Build history of the part. All positions in model axes, mm. Round coordinates to 2 decimals unless told otherwise and drop trailing zeros. Write each loop counter-clockwise with the first axis right and the second up, starting at its lowest first coordinate (ties: lowest second). Pieces come first, ordered by that corner, then holes.
Autodesk Inventor part; units mm, degrees
ref_plane "YZ Plane" through (0, 0, 0) normal (1, 0, 0) x (0, 1, 0)
ref_plane "XZ Plane" through (0, 0, 0) normal (0, 1, 0) x (-1, 0, 0)
ref_plane "XY Plane" through (0, 0, 0) normal (0, 0, 1) x (1, 0, 0)
sketch "Sketch1" plane through (0, 0, 0) normal (0, 1, 0) x (-1, 0, 0)
  line L0 (110, -15) -> (-110, -15)
  line L1 (-110, -15) -> (-110, 15)
  line L2 (-110, 15) -> (110, 15)
  line L3 (110, 15) -> (110, -15)
  line L4 (110, 0) -> (-110, 0) construction
  line L5 (0, -15) -> (0, 15) construction
  point P0 (0, 0)
  point P1 (0, 0)
  dimension "d0" = 220
  dimension "d1" = 30
extrude "Extrusion1" add sketch "Sketch1" along normal blind 15
sketch "Sketch2" plane through (-110, 0, -15) normal (-1, 0, 0) x (0, 0, 1)
  circle A0 centre (5, 7.5) radius 2.5
  line L0 (0, 0) -> (0, 15) construction
  line L1 (0, 7.5) -> (30, 7.5) construction
  line L2 (30, 0) -> (30, 15) construction
  line L3 (15, 0) -> (15, 15) construction
  line L4 (30, 15) -> (0, 15) construction
  circle A1 centre (25, 7.5) radius 2.5
  dimension "d4" = 5
  dimension "d5" = 20
extrude "Extrusion2" cut sketch "Sketch2" against normal blind 8
sketch "Sketch3" plane through (110, 0, 15) normal (1, 0, 0) x (0, 0, -1)
  circle A0 centre (25, 7.5) radius 2.5
  circle A1 centre (5, 7.5) radius 2.5
  point P0 (15, 0)
extrude "Extrusion3" cut sketch "Sketch3" against normal blind 8
properties part number "aux_strut"
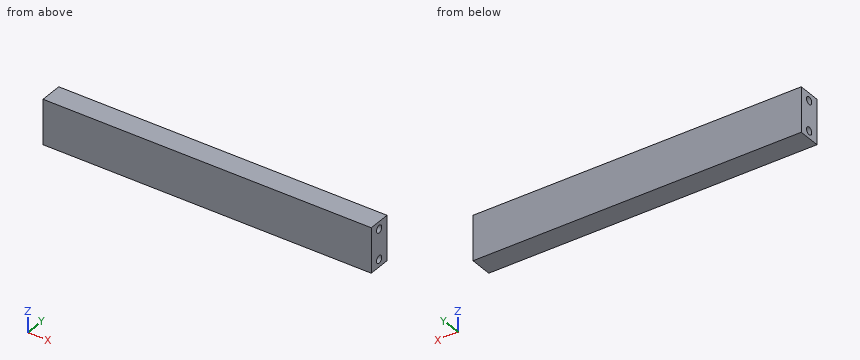
1) Slice it at B-B (y = 7.5). Write the cut outline in (x, z), plus the area to 3 significant figures.
Results:
outline: (-110, -15) - (110, -15) - (110, -12.5) - (102, -12.5) - (102, -7.5) - (110, -7.5) - (110, 7.5) - (102, 7.5) - (102, 12.5) - (110, 12.5) - (110, 15) - (-110, 15) - (-110, 12.5) - (-102, 12.5) - (-102, 7.5) - (-110, 7.5) - (-110, -7.5) - (-102, -7.5) - (-102, -12.5) - (-110, -12.5) - close
area: 6,440 mm2
2) Slice it at A-A (z = -10). Write the cut outline in (x, y).
Results:
outline: (-110, 0) - (110, 0) - (110, 5) - (102, 5) - (102, 10) - (110, 10) - (110, 15) - (-110, 15) - (-110, 10) - (-102, 10) - (-102, 5) - (-110, 5) - close
3) Pin check, flat tips, straight feed: pin 1 Ø2.5 at (y, z) = (7.5, 9.5) entering from -X; pin 2 Ø2.5 at (y, z) = (6.5, 9.5) entering from +X. Stop position of each tip, or through.
Results:
pin 1: stops at x = -102
pin 2: stops at x = 102
4) Wall check: L1, parallel to Y at x = -106.75, z = 10. Give the ranges that are in metal, low to high.
Results:
L1: y = 0 to 5, 10 to 15
